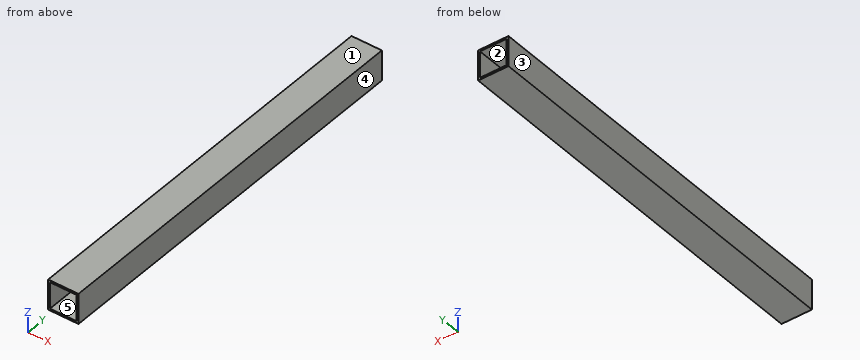
Autodesk Inventor part; units mm, degrees
ref_plane "Work Plane1" through (0, 0, 0) normal (0, 1, 0) x (-1, 0, 0)
ref_plane "YZ Plane" through (0, 0, 0) normal (1, 0, 0) x (0, 1, 0)
ref_plane "XZ Plane" through (0, 0, 0) normal (0, 1, 0) x (-1, 0, 0)
ref_plane "Work Plane1" through (0, 0, 0) normal (0, 1, 0) x (-1, 0, 0)
sketch "Sketch1" plane through (0, 0, 0) normal (0, 1, 0) x (-1, 0, 0)
  line L0 (0, 0) -> (-25.4, 0)
  line L1 (-25.4, 0) -> (-25.4, 25.4)
  line L2 (-25.4, 25.4) -> (0, 25.4)
  line L3 (0, 25.4) -> (0, 0)
  line L4 (-23.8125, 23.8125) -> (-1.5875, 23.8125)
  line L5 (-1.5875, 23.8125) -> (-1.5875, 1.5875)
  line L6 (-1.5875, 1.5875) -> (-23.8125, 1.5875)
  line L7 (-23.8125, 1.5875) -> (-23.8125, 23.8125)
  point P0 (-12.7, 0)
  point P1 (-12.7, 1.5875)
  dimension "d0" = 25.4
  dimension "d1" = 25.4
  dimension "d2" = 1.5875
  dimension "d3" = 1.5875
  dimension "d4" = 1.5875
  dimension "d5" = 1.5875
extrude "Extrusion1" add sketch "Sketch1" along normal blind 330.2
properties part number "54.92Shaft"
The listing builds one solid part. Answer for the finished solid, in the listing's coordinates (mm). Face numbers are marked on the shaded views. A direction names the side the tool comes from. Coordinates: 2 decimals unless noted, no trailing zeros. Loops run counter-clockwise (first coordinate to the right, second up) from the corner with the lowest first, then second, coordinate; pieces in that order, holes last. Notation, with made-up numbers: (84.5, -1.75) -> (123.5, -1.75) arc R23 ccw to (123.5, 28.25) -> close; hole circle Ø10 at (61, -22). An arc over 180 degrees is marked (long way). Return JSON: item names as keys, results as strings. Group by question number.
(1) A cutting plane is placed at A-A on y = 300. Write down the section's boundary in (x, z).
(2) Find the intervals of material crossed by probe 1 along Z at (x, y) = (16, 57), in increasing order. Write a range as from..to.
(3) A cutting plane is placed at C-C on x = 12.75. Write down the section's boundary in (y, z), and give its area (3 significant figures).
(4) Determine the mould class of the marked faces 3, 4 and 5 for opening direction X: released by +X, released by -X, zero draft, split by the parting line, or undercut.
(5) A cutting plane is placed at B-B on z = 7.75. Write down the section's boundary in (x, y).
(6) Given pin 1 Ø4 at (y, z) = (288.5, 6) entering from -X, flat-ended and moving along its own axis, determine where the tip first touches the part or whether it passes through.
(7) Which of the six approach directions +Z, -Z, +X, -X, +Y, -Y give full straight-line access (tool end or side, diameter ignored) to the marked faces 1 and 2?
The answers:
{
 "1": {"outline": "(0, 0) -> (25.4, 0) -> (25.4, 25.4) -> (0, 25.4) -> close; hole (1.59, 1.59) -> (23.81, 1.59) -> (23.81, 23.81) -> (1.59, 23.81) -> close"},
 "2": {"probe 1": "z = 0..1.59, 23.81..25.4"},
 "3": {"outline": "(0, 0) -> (330.2, 0) -> (330.2, 1.59) -> (0, 1.59) -> close; (0, 23.81) -> (330.2, 23.81) -> (330.2, 25.4) -> (0, 25.4) -> close", "area": "1,050 mm^2"},
 "4": {"face 3": "released by -X", "face 4": "released by +X", "face 5": "undercut"},
 "5": {"outline": "(0, 0) -> (1.59, 0) -> (1.59, 330.2) -> (0, 330.2) -> close; (23.81, 0) -> (25.4, 0) -> (25.4, 330.2) -> (23.81, 330.2) -> close"},
 "6": {"pin 1": "stops at x = 0"},
 "7": {"face 1": "+Z, +X, -X, +Y, -Y", "face 2": "+Y, -Y"}
}
